```python
from build123d import *

# Parameters (mm, degrees)
BOX_W              = 40
BOX_H              = 4
BOX_DEPTH          = 38
PAD002_DEPTH       = 3
PAD_DEPTH          = 38
SKETCH001_W        = 15.5
SKETCH001_H        = 3
POCKET_DEPTH       = 7.001
SKETCH002_R        = 12
POCKET001_DEPTH    = 38.001
FILLET_R           = 4
FILLET001_R        = 1
SKETCH003_R        = 1.65
POCKET002_DEPTH    = 7.001
SKETCH004_R        = 3.7
POCKET003_DEPTH    = 3
CHAMFER_SIZE       = 1
CHAMFER001_SIZE    = 1
SKETCH005_W        = 3
SKETCH005_H        = 5
SKETCH005_H_2      = 17
PAD001_DEPTH       = 1
CHAMFER002_SIZE    = 0.99
CHAMFER003_SIZE    = 1
CHAMFER003002_SIZE = 0.4


with BuildPart() as cube:
    # Box → Box (new body)
    with BuildSketch(Plane(origin=(0, 5, 0), x_dir=(1, 0, 0), z_dir=(0, 0, 1))):
        with Locations((20, 2)):
            Rectangle(BOX_W, BOX_H)
    extrude(amount=BOX_DEPTH)


with BuildPart() as body001:
    # Sketch006 → Pad002 (new body)
    with BuildSketch(Plane.XY):
        Polygon((27, -3), (27, 4), (29, 6), (37, 6), (40, 3), (40, -3), (36, -3), (36, 3), (35, 4), (31, 4), (30, 3), (30, -3), align=None)
    extrude(amount=PAD002_DEPTH)


with BuildPart() as body001_1:
    # Body001 placement: moved
    add(body001.part.moved(Location((0, 0, 32))))


with BuildPart() as body002:
    # Body002 base: copy of Body001
    add(body001_1.part)


with BuildPart() as body002_1:
    # Body002 placement: moved
    add(body002.part.moved(Location((0, 0, -8))))


with BuildPart() as body003:
    # Body003 base: copy of Body002
    add(body002_1.part)


with BuildPart() as body003_1:
    # Body003 placement: moved
    add(body003.part.moved(Location((0, 0, -19))))


with BuildPart() as fusion:
    # Body004 base: copy of Body003
    add(body003_1.part)


with BuildPart() as fusion_1:
    # Body004 placement: moved
    add(fusion.part.moved(Location((0, 0, 8))))

    # Fusion: union Body001, Body002, Body003
    add(body001_1.part)
    add(body002_1.part)
    add(body003_1.part)


with BuildPart() as fusion_2:
    # Fusion placement: moved
    add(fusion_1.part.moved(Location((0, -1.5, 0))))


with BuildPart() as chamfer003002:
    # Sketch → Pad (new body)
    with BuildSketch(Plane.XY):
        Polygon((0, 0), (0, 5), (15.5, 5), (15.5, 7), (25, 7), (40, 7), (40, 0), (25, 0), align=None)
    extrude(amount=PAD_DEPTH)

    # Sketch001 (on Face8 of Pad) → Pocket (cut, through all)
    with BuildSketch(Plane.XZ):
        with Locations((7.75, 1.5)):
            Rectangle(SKETCH001_W, SKETCH001_H)
    extrude(amount=-POCKET_DEPTH, mode=Mode.SUBTRACT)

    # Sketch002 (on Face4 of Pocket) → Pocket001 (cut, through all)
    with BuildSketch(Plane.XY.offset(38)):
        with Locations((32.5, -11)):
            Circle(SKETCH002_R)
    extrude(amount=-POCKET001_DEPTH, mode=Mode.SUBTRACT)

    # Fillet
    fillet_edges = [chamfer003002.edges().sort_by_distance(p)[0] for p in [
        (27.704168, 0, 19),
        (37.295832, 0, 19),
    ]]
    fillet(fillet_edges, radius=FILLET_R)

    # Fillet001
    fillet001_edges = [chamfer003002.edges().sort_by_distance(p)[0] for p in [
        (40, 0, 19),
        (40, 7, 19),
    ]]
    fillet(fillet001_edges, radius=FILLET001_R)

    # Sketch003 (on Face12 of Fillet001) → Pocket002 (cut, through all)
    with BuildSketch(Plane.XZ):
        with Locations((7.5, 31)):
            Circle(SKETCH003_R)
        with Locations((7.5, 10)):
            Circle(SKETCH003_R)
    extrude(amount=-POCKET002_DEPTH, mode=Mode.SUBTRACT)

    # Sketch004 (on Face12 of Pocket002) → Pocket003 (cut)
    with BuildSketch(Plane.XZ):
        with Locations((7.5, 31)):
            Circle(SKETCH004_R)
        with Locations((7.5, 10)):
            Circle(SKETCH004_R)
    extrude(amount=-POCKET003_DEPTH, mode=Mode.SUBTRACT)

    # Chamfer
    chamfer_edges = [chamfer003002.edges().sort_by_distance(p)[0] for p in [
        (0, 2.5, 38),
        (0, 2.5, 3),
        (15.5, 2.5, 0),
    ]]
    chamfer(chamfer_edges, length=CHAMFER_SIZE)

    # Chamfer001
    chamfer001_edges = [chamfer003002.edges().sort_by_distance(p)[0] for p in [
        (13, 0, 38),
        (32.5, 1, 0),
    ]]
    chamfer(chamfer001_edges, length=CHAMFER001_SIZE)

    # Sketch005 (on Face4 of Chamfer001) → Pad001 (join)
    with BuildSketch(Plane(origin=(0, 5, 0), x_dir=(-1, 0, 0), z_dir=(0, 1, 0))):
        with Locations((-7.5, 35.5)):
            Rectangle(SKETCH005_W, SKETCH005_H)
        with Locations((-7.5, 20.5)):
            Rectangle(SKETCH005_W, SKETCH005_H_2)
        with Locations((-7.5, 5.5)):
            Rectangle(SKETCH005_W, SKETCH005_H)
    extrude(amount=PAD001_DEPTH)

    # Chamfer002
    chamfer002_edges = [chamfer003002.edges().sort_by_distance(p)[0] for p in [
        (7.5, 6, 29),
        (7.5, 6, 8),
        (7.5, 6, 38),
    ]]
    chamfer(chamfer002_edges, length=CHAMFER002_SIZE)

    # Cut: cut Fusion
    add(fusion_2.part, mode=Mode.SUBTRACT)

    # Cut001: cut Cube
    add(cube.part, mode=Mode.SUBTRACT)

    # Chamfer003
    chamfer003_edges = [chamfer003002.edges().sort_by_distance(p)[0] for p in [
        (40, 1.5, 6.5),
        (40, 1.5, 14.5),
        (40, 1.5, 25.5),
        (40, 1.5, 33.5),
    ]]
    chamfer(chamfer003_edges, length=CHAMFER003_SIZE)

    # Chamfer003002
    chamfer003002_edges = [chamfer003002.edges().sort_by_distance(p)[0] for p in [
        (40, 5, 19),
        (39.5, 5, 0.5),
        (39.5, 5, 37.5),
        (27.75, 5, 0),
        (20, 5, 38),
        (16, 5, 0.5),
        (15.5, 5, 2),
        (0.5, 5, 37.5),
        (8.25, 5, 3),
        (0, 5, 20.5),
        (0.5, 5, 3.5),
        (5.85, 5, 31),
        (5.85, 5, 10),
    ]]
    chamfer(chamfer003002_edges, length=CHAMFER003002_SIZE)


solid = chamfer003002.part
```
Geometry check sheet. Reference: the model listing, model coordinates, mm. A direction names the side the tool comes from. Give positions to 0.01 mm unless a question says otherwise; leave off trailing zeros. Write each loop counter-clockwise with the first axis right and the second up, starting at its lowest first coordinate (ties: lowest second). Pieces come first, ordered by that corner, then holes.
1) Section check A-A, the plane z = 31. Record the boundary of the cut face in (x, y), and give its area (3 significant figures).
2) Section check D-D, the plane z = 19.5. Record the boundary of the cut face in (x, y).
3) Section check B-B, the plane x = 7.5. Record the boundary of the cut face in (y, z), and give its area (3 significant figures).
4) Release check for a two-part mould opening along Z. For faces 5 (the flat face through (16, 2.3, 0.5)), 6 (the flat face through (28, 3.5, 33.5)), 7 (the flat face through (13, 0, 19)), 8 (the flat face through (36, 1, 25)) record: pulls with the +Z half, pulls with the -Z half, needs draft (parallel to the pull), parting line crosses it, or undercut.
5) Section check C-C, the plane x = 15. Record the boundary of the cut face in (y, z), and give its area (3 significant figures).
6) Access from +Z, -Z, +X, -X, +Y, -Y to the whole of each face (thin tool, end or side, straight path). Record for faces 1 (the cylindrical face through (37.351, 0.065, 36.014)), 2 (the flat face through (8, 2, 3)), 3 (the flat face through (35.5, 2, 33.5)), 4 (the flat face through (0.65, 4.803, 37.364)).
7) Material ranges on L1, parallel to Z at x = 7.5, y = 1.6; L2, parallel to Z at x = 7.5, y = 4.1; L3, parallel to Z at x = 35, y = 3.35, recorded low to high.
8) Gauge pin test, flat ends, axial feed: pin 1 (0.5 mm diameter, centred on y = 1, z = 25.5, fed in from +X); pin 2 (6.5 mm diameter, centred on x = 7.5, z = 10, fed in from -Y); pin 3 (4 mm diameter, centred on x = 7.5, z = 31, fed in from +Y). Record the tip position at first contact, or that the pin passes through.
Computed:
1. outline: (0, 0) - (3.8, 0) - (3.8, 3) - (5.85, 3) - (5.85, 4.6) - (5.45, 5) - (0.4, 5) - (0, 4.6) - close; (9.15, 3) - (11.2, 3) - (11.2, 0) - (26.93, 0) arc R4 ccw to (28.32, 0.25) arc R12 cw to (36.68, 0.25) arc R4 ccw to (38.07, 0) - (39, 0) arc R1 ccw to (40, 1) - (40, 4.6) - (39.6, 5) - (9.55, 5) - (9.15, 4.6) - close
1. area: 164 mm2
2. outline: (0, 0) - (26.93, 0) arc R4 ccw to (28.32, 0.25) arc R12 cw to (36.68, 0.25) arc R4 ccw to (38.07, 0) - (39, 0) arc R1 ccw to (40, 1) - (40, 4.6) - (39.6, 5) - (0.4, 5) - (0, 4.6) - close
3. outline: (0, 3) - (4.6, 3) - (5, 3.4) - (5, 7.95) - (4.6, 8.35) - (3, 8.35) - (3, 6.3) - (0, 6.3) - close; (0, 13.7) - (3, 13.7) - (3, 11.65) - (4.6, 11.65) - (5, 12.05) - (5, 28.95) - (4.6, 29.35) - (3, 29.35) - (3, 27.3) - (0, 27.3) - close; (0, 34.7) - (3, 34.7) - (3, 32.65) - (4.6, 32.65) - (5, 33.05) - (5, 37.6) - (4.6, 38) - (1, 38) - (0, 37) - close
3. area: 116 mm2
4. face 5: pulls with the -Z half
4. face 6: undercut
4. face 7: needs draft
4. face 8: undercut
5. outline: (0, 3) - (4.6, 3) - (5, 3.4) - (5, 37.6) - (4.6, 38) - (1, 38) - (0, 37) - close
5. area: 174 mm2
6. face 1: +Z, -Z, -Y
6. face 2: -Z, -X, +Y, -Y
6. face 3: none
6. face 4: +Z, -X, +Y
7. L1: z = 3 to 6.3, 13.7 to 27.3, 34.7 to 38
7. L2: z = 3 to 8.35, 11.65 to 29.35, 32.65 to 38
7. L3: z = 0 to 5, 8 to 13, 16 to 24, 27 to 32, 35 to 38
8. pin 1: stops at x = 36
8. pin 2: stops at y = 3
8. pin 3: stops at y = 4.95
